from build123d import *

# Parameters (mm, degrees)
BOSS_EXTRUDE1_DEPTH = 21
CUT_EXTRUDE1_START  = 21
CUT_EXTRUDE1_DEPTH  = 12


with BuildPart() as part:
    # Sketch1 → Boss-Extrude1 (new body)
    with BuildSketch(Plane.XY):
        with BuildLine():
            ThreePointArc((1.658312395, 2.5), (0, 3), (-1.658312395, 2.5))
            Line((-1.658312395, 2.5), (1.658312395, 2.5))
        make_face()
        with BuildLine():
            Line((1.658312395, 2.5), (-1.658312395, 2.5))
            ThreePointArc((-1.658312395, 2.5), (-1.418637165, -2.643382037), (3, 0))
            ThreePointArc((3, 0), (2.643382037, 1.418637165), (1.658312395, 2.5))
        make_face()
    extrude(amount=BOSS_EXTRUDE1_DEPTH)

    # Sketch1<3> → Cut-Extrude1 (cut)
    with BuildSketch(Plane.XY.offset(CUT_EXTRUDE1_START)):
        Polygon((-26.073564647, 2.5), (-1.658312395, 2.5), (1.658312395, 2.5), (26.073564647, 2.5), (26.073564647, 51.330504504), (-26.073564647, 51.330504504), align=None)
    extrude(amount=-CUT_EXTRUDE1_DEPTH, mode=Mode.SUBTRACT)


solid = part.part
Work out the finished part from the listing and answer in its coordinate system (mm). A direction names the side the tool comes from. Give positions to 0.01 mm unless a question says otherwise; leave off trailing zeros. Loops run counter-clockwise (first coordinate to the right, second up) from the corner with the lowest first, then second, coordinate; pieces in that order, holes last. Notation, with made-up numbers: (-4.75, 66) -> (47.25, 66) arc R19 ccw to (47.25, 73) -> close; hole circle Ø9 at (-8, -35). An arc over 180 degrees is marked (long way). Use a Markdown table: item, result. Add a question column.
1) Each of these flat-tipped pins is pushed along its axis until it touches: P1, Ø1, axis at x = -1, z = 15.5, coming from the +Y side; P2, Ø3, axis at y = -1, z = 11, coming from the -X side. Where does it stop, or does it pass through?
2) The part is cut by section A-A, the plane z = 17.5. Determine the outline of the cut face in (x, y).
3) The part is cut by section C-C, the plane y = 1.15. Determine the outline of the cut face in (x, z), plus the area to 3 significant figures.
4) The part is cut by section B-B, the plane x = 0. Determine the outline of the cut face in (y, z).
5) Consider line 1 along Z through (x, y) = (-0.25, 2.55); line 2 along Y through (x, z) = (-0.7, 6.75); line 3 along Y through (x, z) = (-1.9, 13). Determine where each line is inside the solid, lowest interval first.
6) The part is cut by section D-D, the plane x = 1.1. Determine the outline of the cut face in (y, z), plus the area to 3 significant figures.
7) Which of the six approach directions +Z, -Z, +X, -X, +Y, -Y give full straight-line access (tool end or side, diameter ignored) to faces 1 (the flat face through (0, 0, 0)), 2 (the flat face through (0, 2.5, 15))?
Reported:
| question | item | result |
|---|---|---|
| 1 | P1 | stops at y = 2.5 |
| 1 | P2 | stops at x = -3 |
| 2 | outline | (-1.66, 2.5) arc R3 ccw (long way) to (1.66, 2.5) -> close |
| 3 | outline | (-2.77, 0) -> (2.77, 0) -> (2.77, 21) -> (-2.77, 21) -> close |
| 3 | area | 116 mm^2 |
| 4 | outline | (-3, 0) -> (3, 0) -> (3, 9) -> (2.5, 9) -> (2.5, 21) -> (-3, 21) -> close |
| 5 | line 1 | z = 0 to 9 |
| 5 | line 2 | y = -2.92 to 2.92 |
| 5 | line 3 | y = -2.32 to 2.32 |
| 6 | outline | (-2.79, 0) -> (2.79, 0) -> (2.79, 9) -> (2.5, 9) -> (2.5, 21) -> (-2.79, 21) -> close |
| 6 | area | 114 mm^2 |
| 7 | face 1 | -Z, +X, -X, +Y, -Y |
| 7 | face 2 | +Z, +X, -X, +Y |
